from build123d import *

# Parameters (mm, degrees)
SKETCH1_W           = 70
SKETCH1_H           = 64
BOSS_EXTRUDE1_DEPTH = 10
BOSS_EXTRUDE2_DEPTH = 64
BOSS_EXTRUDE3_DEPTH = 1.3
SKETCH5_W           = 52
SKETCH5_H           = 7
CUT_EXTRUDE1_DEPTH  = 75.042487803
SKETCH6_W           = 4
SKETCH6_H           = 58
CUT_EXTRUDE2_DEPTH  = 79.008268792


with BuildPart() as part:
    # Sketch1 → Boss-Extrude1 (new body)
    with BuildSketch(Plane.XY):
        Rectangle(SKETCH1_W, SKETCH1_H)
    extrude(amount=BOSS_EXTRUDE1_DEPTH)

    # Sketch2 → Boss-Extrude2 (add, through all)
    with BuildSketch(Plane(origin=(0, 32, 0), x_dir=(1, 0, 0), z_dir=(0, 1, 0))):
        Polygon((27.84617358, -12.7), (29.581467698, -12.7), (34.34617358, -10), (30.84617358, -10), (30.84617358, -10.3), (27.84617358, -12), align=None)
    boss_extrude2 = extrude(amount=-BOSS_EXTRUDE2_DEPTH)

    # Mirror1: Boss-Extrude2 across plane
    add(boss_extrude2.mirror(Plane.ZY))

    # Sketch3 → Boss-Extrude3 (add)
    with BuildSketch(Plane.XZ.offset(32)):
        Polygon((-27.84617358, 12), (-27.84617358, 12.7), (27.84617358, 12.7), (27.84617358, 12), (30.84617358, 10.3), (30.84617358, 10), (-30.84617358, 10), (-30.84617358, 10.3), align=None)
    extrude(amount=-BOSS_EXTRUDE3_DEPTH)

    # Sketch5 → Cut-Extrude1 (cut, through all)
    with BuildSketch(Plane(origin=(0, 32, 0), x_dir=(1, 0, 0), z_dir=(0, 1, 0))):
        with Locations((0, -3.5)):
            Rectangle(SKETCH5_W, SKETCH5_H)
    extrude(amount=-CUT_EXTRUDE1_DEPTH, mode=Mode.SUBTRACT)

    # Sketch6 → Cut-Extrude2 (cut, through all)
    with BuildSketch(Plane(origin=(35, 0, 0), x_dir=(0, 0, -1), z_dir=(1, 0, 0))):
        with Locations((-5, 0)):
            Rectangle(SKETCH6_W, SKETCH6_H)
    extrude(amount=-CUT_EXTRUDE2_DEPTH, mode=Mode.SUBTRACT)


solid = part.part
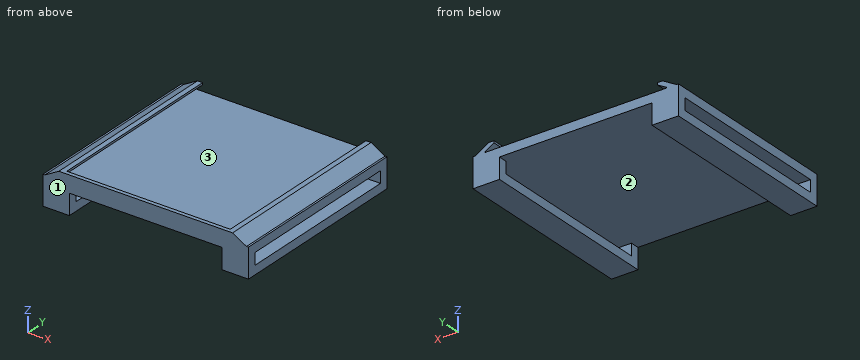
Design review of the part built by this model. Coordinates are the model's own, in mm. Face numbers are marked on the shaded views. Coordinates: 2 decimals unless noted, no trailing zeros. Write each loop counter-clockwise with the first axis right and the second up, starting at its lowest first coordinate (ties: lowest second). Pieces come first, ordered by that corner, then holes. Notation, with made-up numbers: (-9, 56.25) -> (46, 56.25) arc R15 cw to (46, 82.25) -> close; hole circle Ø11 at (15, 76). An arc over 180 degrees is marked (long way). Write each question's results on one line, items separated by ' | '. Start each with the question number.
(1) Take a section at A-A on y = -8.5. Write out the cut boundary in (x, z), and give its area (3 significant figures).
(2) Clearance check with flat-ended pins moving along their axes: P1, Ø2, axis at y = -3, z = 5, coming from the -X side; P2, Ø2, axis at x = 15.5, z = 11.5, coming from the +Y side; P3, Ø8, axis at x = 20.5, y = 20.5, coming from the -Z side; P4, Ø0.6, axis at y = -9.5, z = 12.5, coming from the +X side. State where each tip first meets the part, or that it passes through.
(3) Take a section at B-B on z = 4.25. Write out the cut boundary in (x, y), and give its area (3 significant figures).
(4) Take a section at C-C on x = 10.5. Write out the cut boundary in (y, z), and give its area (3 significant figures).
(5) For line 1 along Y through (x, z) = (28.5, 5.25); line 2 along Z through (x, y) = (27, -27); line 3 along Z through (x, y) = (-28.5, -20), list the stretches that pass through material, from the lowest coordinate up. Write a range as from..to.
(6) The part is to be moulded in two halves that separate along Y. For the marked faces 1, 2 and 3, say which applies: pulls with the +Y half, pulls with the -Y half, needs draft (parallel to the pull), parting line crosses it, or undercut.
Results found:
1) outline: (-35, 0) -> (-26, 0) -> (-26, 3) -> (-35, 3) -> close; (-35, 7) -> (35, 7) -> (35, 10) -> (34.35, 10) -> (29.58, 12.7) -> (27.85, 12.7) -> (27.85, 12) -> (30.85, 10.3) -> (30.85, 10) -> (-30.85, 10) -> (-30.85, 10.3) -> (-27.85, 12) -> (-27.85, 12.7) -> (-29.58, 12.7) -> (-34.35, 10) -> (-35, 10) -> close; (26, 0) -> (35, 0) -> (35, 3) -> (26, 3) -> close | area: 279 mm2
2) P1: passes through | P2: stops at y = -30.7 | P3: stops at z = 7 | P4: stops at x = 30.46
3) outline: (-35, -32) -> (-26, -32) -> (-26, -29) -> (-35, -29) -> close; (-35, 29) -> (-26, 29) -> (-26, 32) -> (-35, 32) -> close; (26, -32) -> (35, -32) -> (35, -29) -> (26, -29) -> close; (26, 29) -> (35, 29) -> (35, 32) -> (26, 32) -> close | area: 108 mm2
4) outline: (-32, 7) -> (32, 7) -> (32, 10) -> (-30.7, 10) -> (-30.7, 12.7) -> (-32, 12.7) -> close | area: 196 mm2
5) line 1: y = -32..-29, 29..32 | line 2: z = 0..3, 7..10 | line 3: z = 0..3, 7..10, 11.63..12.7
6) face 1: pulls with the -Y half | face 2: undercut | face 3: needs draft
